from build123d import *

# Parameters (mm, degrees)
F0_R          = 5
F0_R_2        = 4
F1_DEPTH      = 150
F2_R          = 1
F3_DEPTH      = 5.001
F3_DEPTH_BACK = 5.001
F4_R          = 1
F5_DEPTH      = 5.0010001
F5_DEPTH_BACK = 5.0010001


with BuildPart() as f1:
    # F0 (on Top) → F1 (new body, symmetric)
    with BuildSketch(Plane.XY):
        Circle(F0_R)
        Circle(F0_R_2, mode=Mode.SUBTRACT)
    extrude(amount=F1_DEPTH, both=True)

    # F2 (on Front) → F3 (cut, two sides)
    with BuildSketch(Plane.XZ) as f3_sk:
        with Locations((0, -105)):
            Circle(F2_R)
    extrude(amount=-F3_DEPTH, mode=Mode.SUBTRACT)
    extrude(f3_sk.sketch, amount=F3_DEPTH_BACK, mode=Mode.SUBTRACT)

    # F4 (on Right) → F5 (cut, two sides)
    with BuildSketch(Plane.YZ) as f5_sk:
        with Locations((0, 138)):
            Circle(F4_R)
    extrude(amount=-F5_DEPTH, mode=Mode.SUBTRACT)
    extrude(f5_sk.sketch, amount=F5_DEPTH_BACK, mode=Mode.SUBTRACT)


solid = f1.part
Could you check a few things on this model? Use its own coordinates, in mm. Round coordinates to 2 decimals unless told otherwise and drop trailing zeros. Write each loop counter-clockwise with the first axis right and the second up, starting at its lowest first coordinate (ties: lowest second). Pieces come first, ordered by that corner, then holes. Notation, with made-up numbers: (54.25, -4.75) - (74.25, -4.75) arc R8 ccw to (74.25, 2.25) - close; hole circle Ø4 at (34.5, 42). An arc over 180 degrees is marked (long way). Put each result on its own line as item: value. Start each with the question number.
(1) I want a section at A-A, the plane z = -69.5. Please give me the cut outline in (x, y), plus the area to 3 significant figures.
(2) Will these pins go through, and if not, where does the flat tip stop? pin 1 (4 mm diameter, centred on x = -2.5, y = -2.5, fed in from +Z); pin 2 (1.8 mm diameter, centred on x = 0, z = -105, fed in from +Y); pin 3 (1 mm diameter, centred on x = 4, z = 19, fed in from -Y); pin 4 (2 mm diameter, centred on y = -3, z = 36.5, fed in from -X).
(3) I need wall thicknesses on probe 1 along X at (y, z) = (0, 64); probe 2 along X at (y, z) = (-0.75, 27); probe 3 along Z at (x, y) = (0, 4.8). Which ranges of each line are inside material? Lowest first, please.
(4) Thinking about a two-plate mould opening in X: for faces 1 (the cylindrical face through (-0.867, -3.905, -2.1)), 2 (the cylindrical face through (-1.08, -4.88, 2.1)), which applies, released by +X, released by -X, zero draft, split by the parting line, or undercut?
Here are the results:
1. outline: circle Ø10 at (0, 0); hole circle Ø8 at (0, 0)
1. area: 28.3 mm^2
2. pin 1: stops at z = 150
2. pin 2: passes through
2. pin 3: stops at y = -3.57
2. pin 4: stops at x = -4.58
3. probe 1: x = -5 to -4, 4 to 5
3. probe 2: x = -4.94 to -3.93, 3.93 to 4.94
3. probe 3: z = -150 to -106, -104 to 150
4. face 1: undercut
4. face 2: split by the parting line
